Can you work these out from the model? Positions are in its coordinate system, mm. A direction names the side the tool comes from. Give positions to 0.01 mm unless a question says otherwise; leave off trailing zeros. Write each loop counter-clockwise with the first axis right and the second up, starting at its lowest first coordinate (ties: lowest second). Pieces come first, ordered by that corner, then holes. Notation, with made-up numbers: (42.25, 20) - (87.25, 20) arc R7 cw to (87.25, 29) - close; hole circle Ø5 at (-37.75, -25.75). An arc over 180 degrees is marked (long way). Use a Markdown table: item, result. Add a question column.
```python
from build123d import *

# Parameters (mm, degrees)
F3_W      = 40
F3_H      = 5
F4_DEPTH  = 35.001
F6_D      = 12.1
F9_D      = 3.3
F11_DEPTH = 17.0010001


with BuildPart() as f1:
    # F0 (on Front) → F1 (revolve)
    with BuildSketch(Plane.XZ):
        Polygon((-125, 7.5), (-125, 3.75), (-121.25, 0), (121.25, 0), (125, 3.75), (125, 7.5), (25, 7.5), (25, 10), (-25, 10), (-25, 7.5), align=None)
    revolve(axis=Axis((-80.2068784833, 0, 0), (1, 0, 0)))

    # F3 (on offset) → F4 (cut, through all)
    with BuildSketch(Plane.XY.offset(25)):
        with Locations((0, 9.5)):
            Rectangle(F3_W, F3_H)
        with Locations((0, -9.5)):
            Rectangle(F3_W, F3_H)
    extrude(amount=-F4_DEPTH, mode=Mode.SUBTRACT)

    # F6 (through all)
    with Locations(Plane(origin=(0, 7, 0), x_dir=(-1, 0, 0), z_dir=(0, 1, 0))):
        with Locations((0, 0)):
            Hole(F6_D / 2)

    # F9 (through all)
    with Locations(Plane(origin=(0, 0, -10), x_dir=(1, 0, 0), z_dir=(0, 0, -1))):
        with Locations((0, 0), (-10, 0), (10, 0)):
            Hole(F9_D / 2)

    # F10 (on face) → F11 (cut, through all)
    with BuildSketch(Plane(origin=(0, 7, 0), x_dir=(-1, 0, 0), z_dir=(0, 1, 0))):
        with BuildLine():
            Line((3.4062442661, -5), (13.4062442661, -5))
            Line((13.4062442661, -5), (13.4062442661, 5))
            Line((13.4062442661, 5), (3.4062442661, 5))
            ThreePointArc((3.4062442661, 5), (6.05, 0), (3.4062442661, -5))
        make_face()
        with BuildLine():
            Line((-13.4062442661, 5), (-13.4062442661, -5))
            Line((-13.4062442661, -5), (-3.4062442661, -5))
            ThreePointArc((-3.4062442661, -5), (-6.05, 0), (-3.4062442661, 5))
            Line((-3.4062442661, 5), (-13.4062442661, 5))
        make_face()
    extrude(amount=-F11_DEPTH, mode=Mode.SUBTRACT)


solid = f1.part
```
Q1. Suppose I cut it at B-B (x = -32.5). Please give me the cut outline in (y, z), and give its area (3 significant figures).
Q2. On a 3-axis mill with a long thin cutter (end or side, diameter ignored), from which of +Z, -Z, +X, -X, +Y, -Y can I reach the whole of each face in a straight line? I mean faces 4 (the flat face through (-25, -7, 4)), 5 (the flat face through (25, -7, -4)), 6 (the cylindrical face through (0.85, -1.65, 5.99)). Say none if no direction works.
Q3. Suppose I cut it at A-A (x = 5.5). Please give me the cut outline in (y, z), and give its area (3 significant figures).
Q4. If we mould it in two halves opening along X, with no side actions, what happens to faces 1 (the flat face through (125, 3, -3)), 2 (the cylindrical face through (-0.85, -1.65, -5.99)), 3 (the cylindrical face through (-75.7, -0.33, -7.493))? For each: released by +X, released by -X, zero draft, split by the parting line, or undercut.
Q5. If I drill on probe 1 along Y at (x, z) = (-10, -6.2); probe 2 along Y at (x, z) = (61, 6.5); probe 3 along Y at (x, z) = (-36, -4.5), over which ranges is the centre line in solid material (lowest first)? Write a range as [from, to].
Q6. I'm going to push flat-ended pins straight in: P1, Ø4, axis at x = -12.5, z = 5.5, coming from the -Y side; P2, Ø2, axis at x = 87, y = -5.5, coming from the +Z side; P3, Ø0.9, axis at y = -8, z = 0, coming from the -X side. Where does each tip first touch, or does it pass through?
Derived:
| question | item | result |
|---|---|---|
| 1 | outline | circle Ø15 at (0, 0) |
| 1 | area | 177 mm² |
| 2 | face 4 | -X |
| 2 | face 5 | +X |
| 2 | face 6 | +Y, -Y |
| 3 | outline | (-7, -7.14) arc R10 ccw to (7, -7.14) - (7, -5) - (-7, -5) - close; (-7, 5) - (7, 5) - (7, 7.14) arc R10 ccw to (-7, 7.14) - close |
| 3 | area | 115 mm² |
| 4 | face 1 | released by +X |
| 4 | face 2 | undercut |
| 4 | face 3 | zero draft |
| 5 | probe 1 | [-7, -1.65], [1.65, 7] |
| 5 | probe 2 | [-3.74, 3.74] |
| 5 | probe 3 | [-6, 6] |
| 6 | P1 | y = -7 |
| 6 | P2 | z = 6 |
| 6 | P3 | x = -25 |
